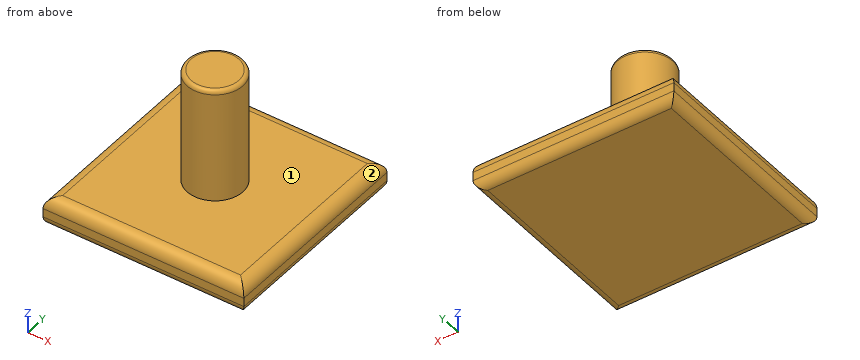
```python
from build123d import *

# Parameters (mm, degrees)
F0_W     = 35
F0_H     = 35
F1_DEPTH = 5
F3_R     = 2
F4_R     = 1.5
F2_R     = 4.85
F5_DEPTH = 20
F6_R     = 0.7


with BuildPart() as f1:
    # F0 (on Top) → F1 (new body)
    with BuildSketch(Plane.XY):
        Rectangle(F0_W, F0_H)
    extrude(amount=-F1_DEPTH)

    # F3
    f3_edges = [f1.edges().sort_by_distance(p)[0] for p in [
        (0, -17.5, 0),
        (-17.5, 0, 0),
        (0, 17.5, 0),
        (17.5, 0, 0),
    ]]
    fillet(f3_edges, radius=F3_R)

    # F4
    f4_edges = [f1.edges().sort_by_distance(p)[0] for p in [
        (0, 17.5, -5),
        (-17.5, 0, -5),
        (0, -17.5, -5),
        (17.5, 0, -5),
    ]]
    fillet(f4_edges, radius=F4_R)

    # F2 (on Top) → F5 (join)
    with BuildSketch(Plane.XY):
        Circle(F2_R)
    extrude(amount=F5_DEPTH)

    # F6
    f6_edges = [f1.edges().sort_by_distance(p)[0] for p in [
        (-4.85, 0, 20),
    ]]
    fillet(f6_edges, radius=F6_R)


solid = f1.part
```
Source: CAD feature listing. Evaluate the final solid. Frame: model axes, mm. Face numbers are marked on the shaded views. A direction names the side the tool comes from. Give positions to 0.01 mm unless a question says otherwise; leave off trailing zeros. Write each loop counter-clockwise with the first axis right and the second up, starting at its lowest first coordinate (ties: lowest second). Pieces come first, ordered by that corner, then holes.
1. Section query A-A (y = 15). Return the cut outline in (x, z), then the cut area to 3 significant figures.
2. Section query C-C (z = 9.5). Return the cut outline in (x, y).
3. Section query D-D (y = 0). Return the cut outline in (x, z), then the cut area to 3 significant figures.
4. Access query for the marked faces 1 and 2. Directions: +Z, -Z, +X, -X, +Y, -Y. A direction counts if a zero-diameter tool reaches every point of the face in a straight line with its end or side. Return the directions, or none.
5. Material intervals for line 1 along Z through (x, y) = (12, 13); line 2 along Y through (x, z) = (8.5, -1); line 3 along X through (y, z) = (12.5, -0.5), sorted ascending.
6. First-contact query: pin 1 (8 mm diameter, centred on x = 9, y = 8.5, fed in from +Z); pin 2 (2 mm diameter, centred on y = 3.5, z = 10, fed in from -X). Flat tips, straight axial feed; report the tip coordinate or a pass-through.
Output values:
1. outline: (-17.5, -3.5) arc R1.5 ccw to (-16, -5) - (16, -5) arc R1.5 ccw to (17.5, -3.5) - (17.5, -2) arc R2 ccw to (15.5, 0) - (-15.5, 0) arc R2 ccw to (-17.5, -2) - close
1. area: 172 mm2
2. outline: circle Ø9.7 at (0, 0)
3. outline: (-17.5, -3.5) arc R1.5 ccw to (-16, -5) - (16, -5) arc R1.5 ccw to (17.5, -3.5) - (17.5, -2) arc R2 ccw to (15.5, 0) - (4.85, 0) - (4.85, 19.3) arc R0.7 ccw to (4.15, 20) - (-4.15, 20) arc R0.7 ccw to (-4.85, 19.3) - (-4.85, 0) - (-15.5, 0) arc R2 ccw to (-17.5, -2) - close
3. area: 366 mm2
4. face 1: +Z
4. face 2: +Z, +X, +Y, -Y
5. line 1: z = -5 to 0
5. line 2: y = -17.23 to 17.23
5. line 3: x = -16.82 to 16.82
6. pin 1: stops at z = 0
6. pin 2: stops at x = -4.16
